Job drawing, mm, ordinate dimensions from the low corner. One solid piece. A direction names the side the tool comes from. Give positions to 0.01 mm unless a question says otherwise; leave off trailing zeros. Write each loop counter-clockwise with the first axis right and the second up, starting at its lowest first coordinate (ties: lowest second). Pieces come first, ordered by that corner, then holes. Notation, with made-up numbers: (-25, 81) -> (17, 81) arc R8 cw to (17, 89) -> close; hole circle Ø11 at (84.25, 64.25). An arc over 180 degrees is marked (long way). Put each result on its own line as item: value. Start each with the question number.
Item 1: Slice it at B-B, the plane z = 20.75. List the corners of the cut face in (x, y), plus the area to 3 significant figures.
Item 2: Slice it at D-D, the plane y = 5.5. List the corners of the cut face in (x, z), plus the area to 3 significant figures.
Item 3: Drill centre lines: line 1 along X through (y, z) = (4.5, 20.75); line 2 along Z through (x, y) = (3.25, 17.75); line 3 along X through (y, z) = (16.55, 20.75). Where is each one in solid material? Low to high.
Item 4: Slice it at C-C, the plane y = 14. List the corners of the cut face in (x, z).
Item 5: Flat gauge pins, fed straight in: pin 1 Ø4 at (x, y) = (5.5, 5.5) entering from -Z; pin 2 Ø1.5 at (x, z) = (7.5, 21.5) entering from -Y; pin 3 Ø3 at (x, z) = (4.5, 21) entering from +Y; pin 4 Ø5 at (x, z) = (5.5, 6) entering from -Y. Where does each tip first touch, or does it go through?
Item 6: Two-plate mould, pull along X, no slides. Class the marked faces 3, 4 and 5: pulls with the +X half, pulls with the -X half, needs draft (parallel to the pull), parting line crosses it, or undercut.
Item 7: Slice it at A-A, the plane x = 5. List the corners of the cut face in (y, z).
Item 8: Tool access for the marked faces 1 and 2: list every direction of +Z, -Z, +X, -X, +Y, -Y with a clear straight run to the whole face (end or side of a thin tool).
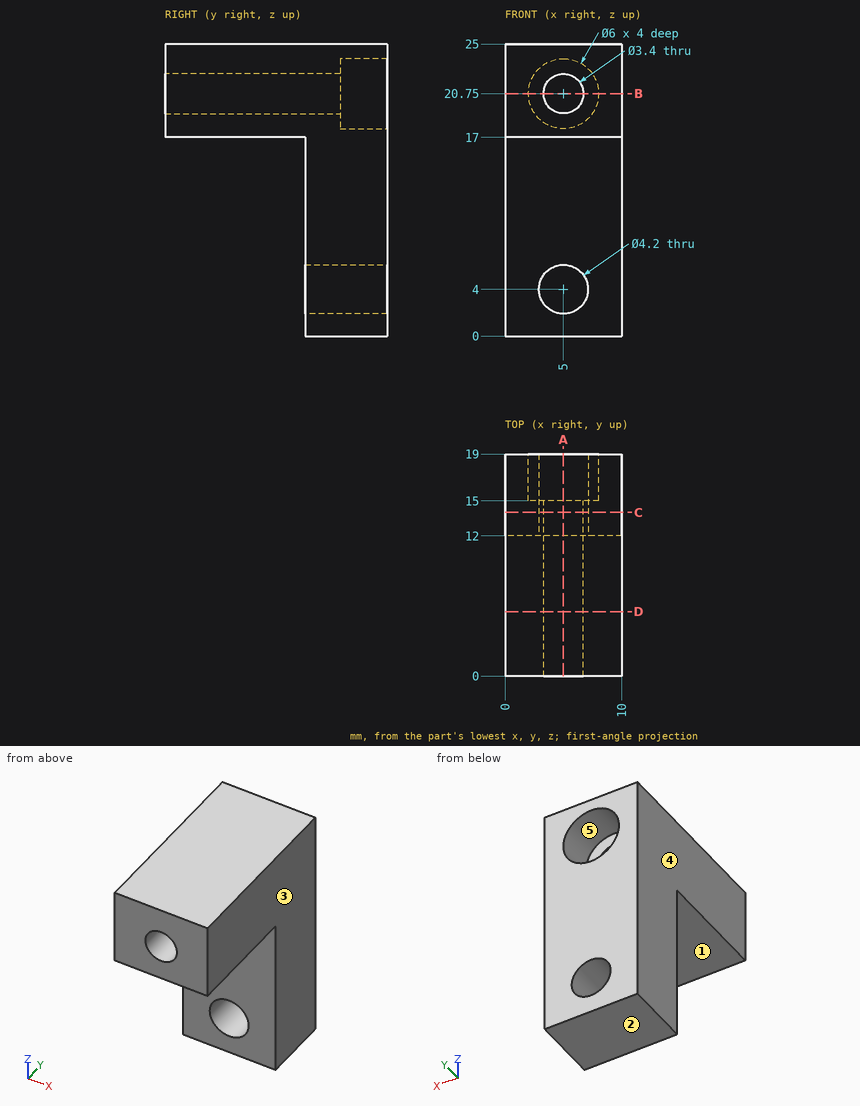
Values follow:
1. outline: (0, 0) -> (3.3, 0) -> (3.3, 15) -> (2, 15) -> (2, 19) -> (0, 19) -> close; (6.7, 0) -> (10, 0) -> (10, 19) -> (8, 19) -> (8, 15) -> (6.7, 15) -> close
1. area: 115 mm2
2. outline: (0, 17) -> (10, 17) -> (10, 25) -> (0, 25) -> close; hole circle Ø3.4 at (5, 20.75)
2. area: 70.9 mm2
3. line 1: 0 to 3.3, 6.7 to 10
3. line 2: 0 to 2.84, 5.16 to 18.31, 23.19 to 25
3. line 3: 0 to 2, 8 to 10
4. outline: (0, 0) -> (10, 0) -> (10, 25) -> (0, 25) -> close; hole circle Ø4.2 at (5, 4); hole circle Ø3.4 at (5, 20.75)
5. pin 1: z = 17
5. pin 2: y = 0
5. pin 3: y = 15
5. pin 4: y = 12
6. face 3: pulls with the +X half
6. face 4: pulls with the -X half
6. face 5: undercut
7. outline: (0, 17) -> (12, 17) -> (12, 6.1) -> (19, 6.1) -> (19, 17.75) -> (15, 17.75) -> (15, 19.05) -> (0, 19.05) -> close; (0, 22.45) -> (15, 22.45) -> (15, 23.75) -> (19, 23.75) -> (19, 25) -> (0, 25) -> close; (12, 0) -> (19, 0) -> (19, 1.9) -> (12, 1.9) -> close
8. face 1: -Z, +X, -X, -Y
8. face 2: -Z, +X, -X, +Y, -Y
